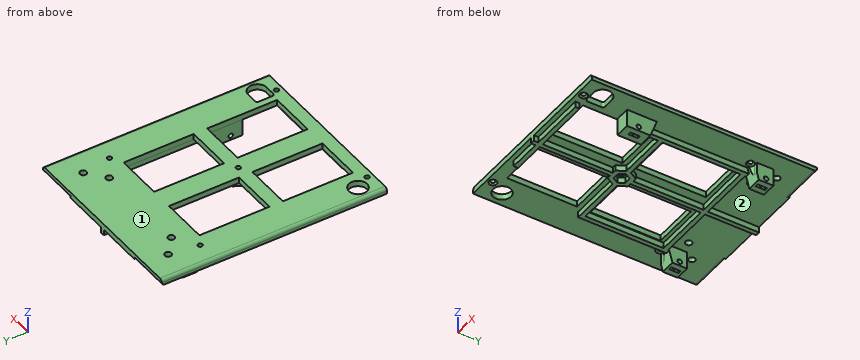
from build123d import *

# Parameters (mm, degrees)
SKETCH1_W                                         = 198.12
SKETCH1_H                                         = 255.039606789
BOSS_EXTRUDE1_DEPTH                               = 6.35
CSK_FOR_8_FLAT_HEAD_MACHINE_SCREW_100_D           = 4.9149
CSK_FOR_8_FLAT_HEAD_MACHINE_SCREW_100_CSINK_D     = 8.4328
CSK_FOR_8_FLAT_HEAD_MACHINE_SCREW_100_CSINK_ANGLE = 100
CUT_EXTRUDE1_REACH                                = 1922.068
SKETCH6_W                                         = 198.12
SKETCH6_H                                         = 10.174402562
F_1_4_CLEARANCE_HOLE1_D                           = 7.14248
FILLET1_R                                         = 3.175
SKETCH9_R                                         = 9.8425
SKETCH9_W                                         = 50.8
SKETCH9_H                                         = 76.2
CUT_EXTRUDE2_DEPTH                                = 1910.907696631
SKETCH10_W                                        = 15.875
SKETCH10_H                                        = 15.875
SKETCH10_H_2                                      = 25.4
BOSS_EXTRUDE2_DEPTH                               = 19.05
BOSS_EXTRUDE3_DEPTH                               = 6.35
DRAFT1_ANGLE                                      = 20
DRAFT2_START                                      = -80.01
DRAFT2_DEPTH                                      = 15.875
DRAFT2_START_2                                    = 64.135
DRAFT2_2_DEPTH                                    = 15.875
F_8_CLEARANCE_HOLE1_REACH                         = 1917.809
F_8_CLEARANCE_HOLE1_BORE_R                        = 2.45745
CUT_EXTRUDE3_START                                = -19.05
CUT_EXTRUDE3_DEPTH                                = 11.526916
CUT_EXTRUDE4_DEPTH                                = 1.651
CUT_EXTRUDE5_REACH                                = 262.327
SKETCH16_W                                        = 25.4
SKETCH16_H                                        = 6.35
CUT_EXTRUDE6_REACH                                = 1911.992
SKETCH17_W                                        = 15.875
SKETCH17_H                                        = 43.91025
FILLET2_START                                     = -100
FILLET2_DEPTH                                     = 46.81875
FILLET2_START_2                                   = 53.18125
FILLET2_2_DEPTH                                   = 46.81875


with BuildPart() as part:
    # Sketch1 → Boss-Extrude1 (new body)
    with BuildSketch(Plane.XY):
        with Locations((0, -1789.981053539)):
            Rectangle(SKETCH1_W, SKETCH1_H)
    extrude(amount=BOSS_EXTRUDE1_DEPTH)

    # CSK for _8 Flat Head Machine Screw _100 (through all)
    with Locations(Plane(origin=(0, 0, 0), x_dir=(-1, 0, 0), z_dir=(0, 0, -1))):
        with Locations((75.59625, -1900.97645438), (-75.59625, -1900.97645438), (75.59625, -1719.49345438), (-75.59625, -1719.49345438), (0, -1810.23495438)):
            CounterSinkHole(CSK_FOR_8_FLAT_HEAD_MACHINE_SCREW_100_D / 2, CSK_FOR_8_FLAT_HEAD_MACHINE_SCREW_100_CSINK_D / 2, counter_sink_angle=CSK_FOR_8_FLAT_HEAD_MACHINE_SCREW_100_CSINK_ANGLE)

    # Sketch6 → Cut-Extrude1 (cut, up to next)
    with BuildSketch(Plane.XY.offset(6.35), mode=Mode.PRIVATE) as cut_extrude1_sk1:
        with Locations((0, -1912.413655653)):
            Rectangle(SKETCH6_W, SKETCH6_H)
    cut_extrude1_tool1 = extrude(cut_extrude1_sk1.sketch, amount=-CUT_EXTRUDE1_REACH, mode=Mode.PRIVATE) & part.part
    add(cut_extrude1_tool1.solids().sort_by_distance((0, -1912.413656, 6.35))[0], mode=Mode.SUBTRACT)

    # 1_4 Clearance Hole1 (through all)
    with Locations(Plane.XY.offset(6.35)):
        with Locations((70.8025, -1687.74345438), (-70.8025, -1687.74345438), (-51.7525, -1703.61845438), (51.7525, -1703.61845438)):
            Hole(F_1_4_CLEARANCE_HOLE1_D / 2)

    # Fillet1
    fillet1_edges = [part.edges().sort_by_distance(p)[0] for p in [
        (-99.06, -1784.893852259, 6.35),
        (99.06, -1784.893852259, 6.35),
    ]]
    fillet(fillet1_edges, radius=FILLET1_R)

    # Sketch9 → Cut-Extrude2 (cut, through all)
    with BuildSketch(Plane(origin=(0, 0, 0), x_dir=(-1, 0, 0), z_dir=(0, 0, -1))):
        with Locations((83.82, -1885.73645438)):
            Circle(SKETCH9_R)
        with Locations((-37.798125, -1855.60570438)):
            Rectangle(SKETCH9_W, SKETCH9_H)
        with Locations((37.798125, -1855.60570438)):
            Rectangle(SKETCH9_W, SKETCH9_H)
        with Locations((37.798125, -1764.86420438)):
            Rectangle(SKETCH9_W, SKETCH9_H)
        with Locations((-37.798125, -1764.86420438)):
            Rectangle(SKETCH9_W, SKETCH9_H)
        with BuildLine():
            Line((-83.82, -1875.789551383), (-72.8191921, -1875.789551383))
            ThreePointArc((-72.8191921, -1875.789551383), (-71.023140876, -1876.533500159), (-70.2791921, -1878.329551383))
            Line((-70.2791921, -1878.329551383), (-70.2791921, -1893.143357377))
            ThreePointArc((-70.2791921, -1893.143357377), (-71.023140876, -1894.939408601), (-72.8191921, -1895.683357377))
            Line((-72.8191921, -1895.683357377), (-83.82, -1895.683357377))
            ThreePointArc((-83.82, -1895.683357377), (-93.766902997, -1885.73645438), (-83.82, -1875.789551383))
        make_face()
    extrude(amount=-CUT_EXTRUDE2_DEPTH, mode=Mode.SUBTRACT)

    # Sketch10 → Boss-Extrude2 (add)
    with BuildSketch(Plane(origin=(0, 0, 0), x_dir=(-1, 0, 0), z_dir=(0, 0, -1))):
        with Locations((-72.0725, -1705.323750137)):
            Rectangle(SKETCH10_W, SKETCH10_H)
        with Locations((72.0725, -1843.82645438)):
            Rectangle(SKETCH10_W, SKETCH10_H_2)
        with Locations((72.0725, -1705.323750137)):
            Rectangle(SKETCH10_W, SKETCH10_H)
        with Locations((-72.0725, -1843.82645438)):
            Rectangle(SKETCH10_W, SKETCH10_H_2)
    extrude(amount=BOSS_EXTRUDE2_DEPTH)

    # Sketch11 → Boss-Extrude3 (add)
    with BuildSketch(Plane(origin=(0, 0, 0), x_dir=(-1, 0, 0), z_dir=(0, 0, -1))):
        Polygon((-64.135, -1718.020391975), (-64.135, -1713.261250137), (-68.8975, -1713.261250137), (-68.8975, -1831.12645438), (-64.135, -1831.12645438), (-64.135, -1812.61620438), (-11.456794404, -1812.61620438), (-6.415804866, -1821.34745438), (-2.38125, -1821.34745438), (-2.38125, -1897.67445438), (-64.135, -1897.67445438), (-64.135, -1902.449516786), (-2.38125, -1902.449516786), (-2.38125, -1907.32645438), (2.38125, -1907.32645438), (2.38125, -1902.449516786), (64.135, -1902.449516786), (64.135, -1897.67445438), (2.38125, -1897.67445438), (2.38125, -1821.34745438), (6.415804866, -1821.34745438), (11.456794404, -1812.61620438), (64.135, -1812.61620438), (64.135, -1831.12645438), (68.8975, -1831.12645438), (68.8975, -1713.261250137), (64.135, -1713.261250137), (64.135, -1718.020391975), (2.38125, -1718.020391975), (2.38125, -1662.461250145), (-2.38125, -1662.461250145), (-2.38125, -1718.020391975), align=None)
        Polygon((-5.95753309, -1812.61620438), (-7.332348419, -1810.23495438), (-5.95753309, -1807.85370438), (-3.666174209, -1803.88495438), (3.666174209, -1803.88495438), (7.332348419, -1810.23495438), (3.666174209, -1816.58495438), (-3.666174209, -1816.58495438), align=None, mode=Mode.SUBTRACT)
        Polygon((-64.135, -1807.85370438), (-64.135, -1722.79545438), (-2.38125, -1722.79545438), (-2.38125, -1799.12245438), (-6.415804866, -1799.12245438), (-11.456794404, -1807.85370438), align=None, mode=Mode.SUBTRACT)
        Polygon((64.135, -1807.85370438), (11.456794404, -1807.85370438), (6.415804866, -1799.12245438), (2.38125, -1799.12245438), (2.38125, -1722.79545438), (64.135, -1722.79545438), align=None, mode=Mode.SUBTRACT)
    extrude(amount=BOSS_EXTRUDE3_DEPTH)

    # Draft1
    draft1_faces = [part.faces().sort_by_distance(p)[0] for p in [
        (72.689861111, -1831.12645438, -10.230555556),
        (-72.689861111, -1831.12645438, -10.230555556),
    ]]
    draft(draft1_faces, Plane(origin=(0, 0, -19.05), x_dir=(-1, 0, 0), z_dir=(0, 0, -1)), DRAFT1_ANGLE)

    # Draft2: read off the stored shape, not the designer's step
    # Draft2 outline → Draft2 (add)
    with BuildSketch(Plane.YZ.offset(DRAFT2_START)):
        Polygon((-1718.365682253, 0), (-1713.261250137, -19.05), (-1713.261250137, 0), align=None)
    extrude(amount=DRAFT2_DEPTH)

    # Draft2 2 outline → Draft2 2 (add)
    with BuildSketch(Plane.YZ.offset(DRAFT2_START_2)):
        Polygon((-1718.365682253, 0), (-1713.261250137, -19.05), (-1713.261250137, 0), align=None)
    extrude(amount=DRAFT2_2_DEPTH)

    # 8 Clearance Hole1 bore → 8 Clearance Hole1 (cut, up to next)
    with BuildSketch(Plane(origin=(80.01, 0, 0), x_dir=(0, 0, -1), z_dir=(1, 0, 0)), mode=Mode.PRIVATE) as f_8_clearance_hole1_sk1:
        with Locations((14.2875, -1843.82645438)):
            Circle(F_8_CLEARANCE_HOLE1_BORE_R)
    f_8_clearance_hole1_tool1 = extrude(f_8_clearance_hole1_sk1.sketch, amount=-F_8_CLEARANCE_HOLE1_REACH, mode=Mode.PRIVATE) & part.part
    # 8 Clearance Hole1 bore → 8 Clearance Hole1 (cut, up to next)
    with BuildSketch(Plane(origin=(80.01, 0, 0), x_dir=(0, 0, -1), z_dir=(1, 0, 0)), mode=Mode.PRIVATE) as f_8_clearance_hole1_sk2:
        with Locations((14.2875, -1705.323750137)):
            Circle(F_8_CLEARANCE_HOLE1_BORE_R)
    f_8_clearance_hole1_tool2 = extrude(f_8_clearance_hole1_sk2.sketch, amount=-F_8_CLEARANCE_HOLE1_REACH, mode=Mode.PRIVATE) & part.part
    f_8_clearance_hole1_1 = f_8_clearance_hole1_tool1.solids().sort_by_distance((80.01, -1843.826454, -14.2875))[0]
    add(f_8_clearance_hole1_1, mode=Mode.SUBTRACT)
    f_8_clearance_hole1_2 = f_8_clearance_hole1_tool2.solids().sort_by_distance((80.01, -1705.32375, -14.2875))[0]
    add(f_8_clearance_hole1_2, mode=Mode.SUBTRACT)
    f_8_clearance_hole1 = f_8_clearance_hole1_1 + f_8_clearance_hole1_2  # 8 Clearance Hole1 as one shape, for the pattern or mirror that repeats it

    # Sketch14 → Cut-Extrude3 (cut)
    with BuildSketch(Plane(origin=(0, 0, -19.05), x_dir=(-1, 0, 0), z_dir=(0, 0, -1)).offset(CUT_EXTRUDE3_START)):
        with BuildLine():
            Line((75.59625, -1715.27705438), (80.01, -1715.27705438))
            Line((80.01, -1715.27705438), (80.01, -1723.70985438))
            Line((80.01, -1723.70985438), (75.59625, -1723.70985438))
            ThreePointArc((75.59625, -1723.70985438), (71.37985, -1719.49345438), (75.59625, -1715.27705438))
        make_face()
        with BuildLine():
            Line((-80.01, -1723.70985438), (-75.59625, -1723.70985438))
            ThreePointArc((-75.59625, -1723.70985438), (-71.37985, -1719.49345438), (-75.59625, -1715.27705438))
            Line((-75.59625, -1715.27705438), (-80.01, -1715.27705438))
            Line((-80.01, -1715.27705438), (-80.01, -1723.70985438))
        make_face()
    extrude(amount=CUT_EXTRUDE3_DEPTH, mode=Mode.SUBTRACT)

    # Sketch15 → Cut-Extrude4 (cut, symmetric)
    with BuildSketch(Plane.ZY.offset(-72.0725)):
        Polygon((-9.7917, -1707.919401478), (-9.7917, -1702.728098797), (-14.2875, -1700.132447457), (-19.05, -1700.132447457), (-19.05, -1710.515052818), (-14.2875, -1710.515052818), align=None)
        Polygon((-19.05, -1838.6351517), (-14.2875, -1838.6351517), (-9.7917, -1841.23080304), (-9.7917, -1846.42210572), (-14.2875, -1849.01775706), (-19.05, -1849.01775706), align=None)
    cut_extrude4 = extrude(amount=CUT_EXTRUDE4_DEPTH, both=True, mode=Mode.SUBTRACT)

    # Mirror1: 8 Clearance Hole1, Cut-Extrude4 across plane
    add(f_8_clearance_hole1.mirror(Plane(origin=(0, 0, 0), x_dir=(0, 0, 1), z_dir=(1, 0, 0))), mode=Mode.SUBTRACT)
    add(cut_extrude4.mirror(Plane(origin=(0, 0, 0), x_dir=(0, 0, 1), z_dir=(1, 0, 0))), mode=Mode.SUBTRACT)

    # Sketch16 → Cut-Extrude5 (cut, up to next)
    with BuildSketch(Plane.XZ.offset(1902.449516786), mode=Mode.PRIVATE) as cut_extrude5_sk1:
        with Locations((-51.435, -3.175)):
            Rectangle(SKETCH16_W, SKETCH16_H)
    cut_extrude5_tool1 = extrude(cut_extrude5_sk1.sketch, amount=-CUT_EXTRUDE5_REACH, mode=Mode.PRIVATE) & part.part
    add(cut_extrude5_tool1.solids().sort_by_distance((-51.435, -1902.449517, -3.175))[0], mode=Mode.SUBTRACT)

    # Sketch17 → Cut-Extrude6 (cut, up to next)
    with BuildSketch(Plane(origin=(0, 0, 0), x_dir=(-1, 0, 0), z_dir=(0, 0, -1)), mode=Mode.PRIVATE) as cut_extrude6_sk1:
        with Locations((72.0725, -1834.57132938)):
            Rectangle(SKETCH17_W, SKETCH17_H)
    cut_extrude6_tool1 = extrude(cut_extrude6_sk1.sketch, amount=CUT_EXTRUDE6_REACH, mode=Mode.PRIVATE) & part.part
    add(cut_extrude6_tool1.solids().sort_by_distance((-72.0725, -1834.571329, 0))[0], mode=Mode.SUBTRACT)

    # Fillet2: read off the stored shape, not the designer's step
    # Fillet2 outline → Fillet2 (cut)
    with BuildSketch(Plane.YZ.offset(FILLET2_START)):
        with BuildLine():
            ThreePointArc((-1662.461250145, 3.175), (-1663.391186115, 0.92993597), (-1665.636250145, 0))
            Line((-1665.636250145, 0), (-1662.461250145, 0))
            Line((-1662.461250145, 0), (-1662.461250145, 3.175))
        make_face()
    extrude(amount=FILLET2_DEPTH, mode=Mode.SUBTRACT)

    # Fillet2 2 outline → Fillet2 2 (cut)
    with BuildSketch(Plane.YZ.offset(FILLET2_START_2)):
        with BuildLine():
            ThreePointArc((-1662.461250145, 3.175), (-1663.391186115, 0.92993597), (-1665.636250145, 0))
            Line((-1665.636250145, 0), (-1662.461250145, 0))
            Line((-1662.461250145, 0), (-1662.461250145, 3.175))
        make_face()
    extrude(amount=FILLET2_2_DEPTH, mode=Mode.SUBTRACT)


solid = part.part
Can you work these out from the model? Positions are in its coordinate system, mm. Face numbers are marked on the shaded views. Coordinates: 2 decimals unless noted, no trailing zeros. Order: outer loops, then holes, each group sorted by start corner. A loop starts at its lowest first (then second) coordinate and runs counter-clockwise, first axis right, second up. Notation, with made-up numbers: M 12,11.5 L 38,11.5 A19 cw 38,30.5 Z; hole C 48,76.25 d8. An arc over 180 degrees is marked long. Write item = value, one per line.
(1) Suppose I cut it at C-C on y = -1759.5. State how many separate pieces and enclosed holes the cut face has, plus the area to 3 significant figures.
Results are:
separate_pieces = 3
enclosed_holes = 0
area = 699 mm2
(2) If we mould it in two halves opening along X, with no side actions, what happens to the marked faces 1 and 2? For each: pulls with the +X half, pulls with the -X half, needs draft (parallel to the pull), parting line crosses it, or undercut.
Results are:
face_1 = needs draft
face_2 = undercut
(3) For pin 1 Ø18.5 at (x, y) = (23, -1778) entering from -Z; pin 2 Ø3 at (y, z) = (-1781.5, -5.5) entering from +X; pin 3 Ø2.5 at (y, z) = (-1901, -3.5) entering from -X (3 decimals); pin 4 Ø6 at (y, z) = (-1787.5, -4) entering from -X, each with a flat end and sliding along its axis, tell me the tip position at first contact or that it passes through.
Results are:
pin_1 = through
pin_2 = 68.9
pin_3 = -38.735
pin_4 = -68.9
(4) I need wall thicknesses on line 1 along Y through (x, z) = (29.5, -5); line 2 along X through (y, z) = (-1745, -2.75) (1 decimal); line 3 along Y through (x, z) = (8, -0.75). Which ranges of each line are inside material? Lowest first, please. Write a range as [from, to].
Results are:
line_1 = [-1902.45, -1897.67], [-1812.62, -1807.85], [-1722.8, -1718.02]
line_2 = [-68.9, -64.1], [-2.4, 2.4], [64.1, 68.9]
line_3 = [-1902.45, -1897.67], [-1818.6, -1801.87], [-1722.8, -1718.02]
(5) Suppose I cut it at A-A on x = -83.82. Please give me the cut outline in (y, z) (3 decimals), plus the area to 3 significant figures.
Results are:
outline = M -1907.326,0 L -1895.579,0 L -1895.579,6.35 L -1907.326,6.35 Z; M -1875.894,0 L -1665.636,0 A3.175 ccw -1662.461,3.175 L -1662.461,6.35 L -1875.894,6.35 Z
area = 1,430 mm2
(6) Suppose I cut it at B-B on x = -17. Please give me the cut outline in (y, z).
Results are:
outline = M -1907.33,0 L -1902.45,0 L -1902.45,-6.35 L -1897.67,-6.35 L -1897.67,0 L -1893.71,0 L -1893.71,6.35 L -1907.33,6.35 Z; M -1817.51,0 L -1812.62,0 L -1812.62,-6.35 L -1807.85,-6.35 L -1807.85,0 L -1802.96,0 L -1802.96,6.35 L -1817.51,6.35 Z; M -1726.76,0 L -1722.8,0 L -1722.8,-6.35 L -1718.02,-6.35 L -1718.02,0 L -1662.46,0 L -1662.46,6.35 L -1726.76,6.35 Z
